Build history of the part. All positions in model axes, mm. Face numbers are marked on the shaded views. A direction names the side the tool comes from. Give positions to 0.01 mm unless a question says otherwise; leave off trailing zeros. Answer as a JSON object with one key per item and string values. Group by question number.
1. 3-axis set-ups, long thin cutter, end or side, ignore diameter. For the marked faces 1 and 2: which of +Z, -Z, +X, -X, +Y, -Y reach the whole face in a straight line?
2. Drop flat-ended pins along their axis: pin 1 Ø2 at (x, y) = (24.5, -20) entering from +Z; pin 2 Ø1 at (y, z) = (16.5, 3) entering from -X; pin 3 Ø12.5 at (x, y) = (-5, 0) entering from +Z. Give the stop position or say it passes through.
3. Drill centre lines: line 1 along Z through (x, y) = (-52.5, 20); line 2 along Z through (x, y) = (25, 33); line 3 along X through (y, z) = (-47, 3.5). Where is each one in solid material? Low to high. Write a range as [from, to].
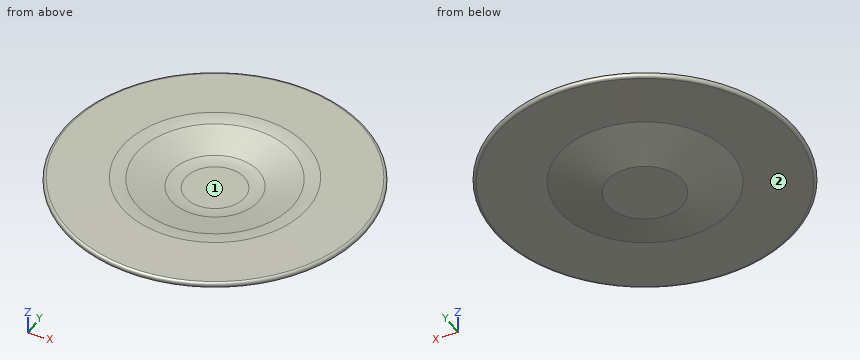
from build123d import *

# Parameters (mm, degrees)
F3_R = 25.4


with BuildPart() as f2:
    # F0 (on Front) → F2 (revolve)
    with BuildSketch(Plane.XZ):
        with BuildLine():
            Line((35.242144, 4.75648), (15.238293, 0))
            Line((15.238293, 0), (0, 0))
            Line((0, 0), (0, -2.286))
            Line((0, -2.286), (15.506336, -2.286))
            Line((15.506336, -2.286), (35.506643, 2.469638))
            Line((35.506643, 2.469638), (61.135289, 2.389061))
            ThreePointArc((61.135289, 2.389061), (62.281877, 3.528461), (61.142476, 4.675049))
            Line((61.142476, 4.675049), (35.242144, 4.75648))
        make_face()
    revolve(axis=Axis((0, 0, 4.155044), (0, 0, 1)))

    # F3
    f3_edges = [f2.edges().sort_by_distance(p)[0] for p in [
        (-35.242144, 0, 4.75648),
        (-15.238293, 0, 0),
    ]]
    fillet(f3_edges, radius=F3_R)


solid = f2.part
Established:
{
 "1": {"face 1": "+Z", "face 2": "-Z"},
 "2": {"pin 1": "stops at z = 4.13", "pin 2": "stops at x = -60.14", "pin 3": "stops at z = 0"},
 "3": {"line 1": "z = [2.4, 4.69]", "line 2": "z = [2.45, 4.74]", "line 3": "x = [-40.87, 40.87]"}
}
